For this review, take the finished solid that the model builds, in its own axes (mm). Coordinates: 2 decimals unless noted, no trailing zeros. Write each loop counter-clockwise with the first axis right and the second up, starting at its lowest first coordinate (ties: lowest second). Pieces come first, ordered by that corner, then holes. Notation, with made-up numbers: (23, -24) - (70, -24) arc R24 ccw to (70, 2) - close; hole circle Ø9 at (28, 35.5). An arc over 180 degrees is marked (long way). Write each question's results on one line, items separated by ' | '.
from build123d import *

# Parameters (mm, degrees)
SKIZZE1_R                       = 17.5
SKIZZE1_R_2                     = 2.2
SKIZZE1_R_3                     = 1.7
SKIZZE1_R_4                     = 2.05
AUFSATZ_LINEAR_AUSTRAGEN1_DEPTH = 2.5


with BuildPart() as part:
    # Skizze1 → Aufsatz-Linear austragen1 (new body)
    with BuildSketch(Plane.XY):
        with BuildLine():
            Line((9.914391914, -80), (9.914391914, 0))
            Line((9.914391914, 0), (9.914391914, 8))
            ThreePointArc((9.914391914, 8), (10.500178351, 9.414213562), (11.914391914, 10))
            Line((11.914391914, 10), (108.085608086, 10))
            ThreePointArc((108.085608086, 10), (109.499821649, 9.414213562), (110.085608086, 8))
            Line((110.085608086, 8), (110.085608086, 0))
            Line((110.085608086, 0), (110.085608086, -80))
            Line((110.085608086, -80), (110.085608086, -88))
            ThreePointArc((110.085608086, -88), (109.499821649, -89.414213562), (108.085608086, -90))
            Line((108.085608086, -90), (11.914391914, -90))
            ThreePointArc((11.914391914, -90), (10.500178351, -89.414213562), (9.914391914, -88))
            Line((9.914391914, -88), (9.914391914, -80))
        make_face()
        with Locations((60, -40)):
            Circle(SKIZZE1_R, mode=Mode.SUBTRACT)
        with Locations((35, -40)):
            Circle(SKIZZE1_R_2, mode=Mode.SUBTRACT)
        with Locations((50, -85)):
            Circle(SKIZZE1_R_3, mode=Mode.SUBTRACT)
        with Locations((24.914391914, -40)):
            Circle(SKIZZE1_R_4, mode=Mode.SUBTRACT)
        with Locations((40, -85)):
            Circle(SKIZZE1_R_3, mode=Mode.SUBTRACT)
        with Locations((95.085608086, -85)):
            Circle(SKIZZE1_R_3, mode=Mode.SUBTRACT)
        with Locations((24.914391914, -85)):
            Circle(SKIZZE1_R_3, mode=Mode.SUBTRACT)
        with Locations((14.914391914, -85)):
            Circle(SKIZZE1_R_3, mode=Mode.SUBTRACT)
        with Locations((105.085608086, -85)):
            Circle(SKIZZE1_R_3, mode=Mode.SUBTRACT)
        with Locations((40, 5)):
            Circle(SKIZZE1_R_3, mode=Mode.SUBTRACT)
        with Locations((50, 5)):
            Circle(SKIZZE1_R_3, mode=Mode.SUBTRACT)
        with Locations((70, 5)):
            Circle(SKIZZE1_R_3, mode=Mode.SUBTRACT)
        with Locations((80, 5)):
            Circle(SKIZZE1_R_3, mode=Mode.SUBTRACT)
        with Locations((95.085608086, 5)):
            Circle(SKIZZE1_R_3, mode=Mode.SUBTRACT)
        with Locations((105.085608086, 5)):
            Circle(SKIZZE1_R_3, mode=Mode.SUBTRACT)
        with Locations((80, -85)):
            Circle(SKIZZE1_R_3, mode=Mode.SUBTRACT)
        with Locations((95.085608086, -40)):
            Circle(SKIZZE1_R_4, mode=Mode.SUBTRACT)
        with Locations((70, -85)):
            Circle(SKIZZE1_R_3, mode=Mode.SUBTRACT)
        with Locations((85, -40)):
            Circle(SKIZZE1_R_2, mode=Mode.SUBTRACT)
        with Locations((24.914391914, 5)):
            Circle(SKIZZE1_R_3, mode=Mode.SUBTRACT)
        with Locations((14.914391914, 5)):
            Circle(SKIZZE1_R_3, mode=Mode.SUBTRACT)
        Polygon((101.462722804, -76.748846085), (103.274165445, -79.886356775), (106.897050727, -79.886356775), (108.708493369, -76.748846085), (106.897050727, -73.611335396), (103.274165445, -73.611335396), align=None, mode=Mode.SUBTRACT)
        Polygon((33.107285571, -56.381153914), (31.300179229, -53.251153914), (33.107285571, -50.121153914), (36.721498256, -50.121153914), (38.528604599, -53.251153914), (36.721498256, -56.381153914), align=None, mode=Mode.SUBTRACT)
        Polygon((18.537277196, -3.251153914), (16.725834555, -0.113643225), (13.102949273, -0.113643225), (11.291506631, -3.251153914), (13.102949273, -6.388664604), (16.725834555, -6.388664604), align=None, mode=Mode.SUBTRACT)
        Polygon((38.528604599, -3.251153914), (36.721498256, -0.121153914), (33.107285571, -0.121153914), (31.300179229, -3.251153914), (33.107285571, -6.381153914), (36.721498256, -6.381153914), align=None, mode=Mode.SUBTRACT)
        Polygon((18.528604599, -26.674423043), (16.721498256, -23.544423043), (13.107285571, -23.544423043), (11.300179229, -26.674423043), (13.107285571, -29.804423043), (16.721498256, -29.804423043), align=None, mode=Mode.SUBTRACT)
        Polygon((31.300179229, -26.748846085), (33.107285571, -29.878846085), (36.721498256, -29.878846085), (38.528604599, -26.748846085), (36.721498256, -23.618846085), (33.107285571, -23.618846085), align=None, mode=Mode.SUBTRACT)
        Polygon((16.721498256, -50.195576957), (18.528604599, -53.325576957), (16.721498256, -56.455576957), (13.107285571, -56.455576957), (11.300179229, -53.325576957), (13.107285571, -50.195576957), align=None, mode=Mode.SUBTRACT)
        Polygon((36.721498256, -73.618846085), (38.528604599, -76.748846085), (36.721498256, -79.878846085), (33.107285571, -79.878846085), (31.300179229, -76.748846085), (33.107285571, -73.618846085), align=None, mode=Mode.SUBTRACT)
        Polygon((16.725834555, -73.611335396), (18.537277196, -76.748846085), (16.725834555, -79.886356775), (13.102949273, -79.886356775), (11.291506631, -76.748846085), (13.102949273, -73.611335396), align=None, mode=Mode.SUBTRACT)
        Polygon((81.471395401, -76.748846085), (83.278501744, -79.878846085), (86.892714429, -79.878846085), (88.699820771, -76.748846085), (86.892714429, -73.618846085), (83.278501744, -73.618846085), align=None, mode=Mode.SUBTRACT)
        Polygon((101.471395401, -53.325576957), (103.278501744, -56.455576957), (106.892714429, -56.455576957), (108.699820771, -53.325576957), (106.892714429, -50.195576957), (103.278501744, -50.195576957), align=None, mode=Mode.SUBTRACT)
        Polygon((88.699820771, -53.251153914), (86.892714429, -50.121153914), (83.278501744, -50.121153914), (81.471395401, -53.251153914), (83.278501744, -56.381153914), (86.892714429, -56.381153914), align=None, mode=Mode.SUBTRACT)
        Polygon((86.892714429, -23.618846085), (88.699820771, -26.748846085), (86.892714429, -29.878846085), (83.278501744, -29.878846085), (81.471395401, -26.748846085), (83.278501744, -23.618846085), align=None, mode=Mode.SUBTRACT)
        Polygon((103.278501744, -29.804423043), (101.471395401, -26.674423043), (103.278501744, -23.544423043), (106.892714429, -23.544423043), (108.699820771, -26.674423043), (106.892714429, -29.804423043), align=None, mode=Mode.SUBTRACT)
        Polygon((83.278501744, -6.381153914), (81.471395401, -3.251153914), (83.278501744, -0.121153914), (86.892714429, -0.121153914), (88.699820771, -3.251153914), (86.892714429, -6.381153914), align=None, mode=Mode.SUBTRACT)
        Polygon((103.274165445, -6.388664604), (101.462722804, -3.251153914), (103.274165445, -0.113643225), (106.897050727, -0.113643225), (108.708493369, -3.251153914), (106.897050727, -6.388664604), align=None, mode=Mode.SUBTRACT)
    extrude(amount=AUFSATZ_LINEAR_AUSTRAGEN1_DEPTH)


solid = part.part
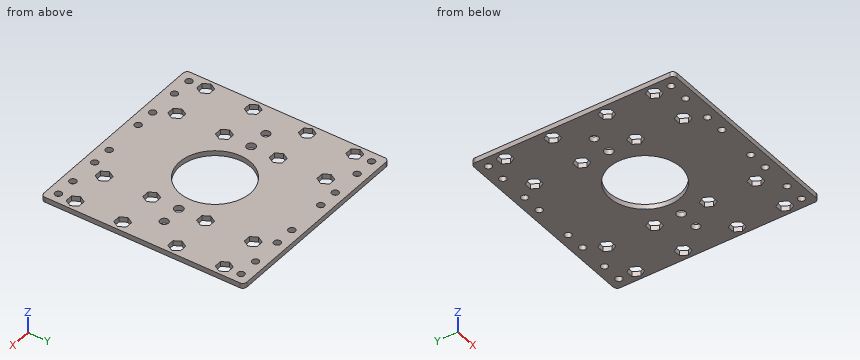
Q1. Take a section at D-D on x = 25. State the section outline as (y, z) points.
Results found:
outline: (-90, 0) - (-86.7, 0) - (-86.7, 2.5) - (-90, 2.5) - close; (-83.3, 0) - (-42.05, 0) - (-42.05, 2.5) - (-83.3, 2.5) - close; (-37.95, 0) - (3.3, 0) - (3.3, 2.5) - (-37.95, 2.5) - close; (6.7, 0) - (10, 0) - (10, 2.5) - (6.7, 2.5) - close
Q2. Take a section at B-B on x = 60. State the section outline as (y, z) points.
Results found:
outline: (-90, 0) - (-57.5, 0) - (-57.5, 2.5) - (-90, 2.5) - close; (-22.5, 0) - (10, 0) - (10, 2.5) - (-22.5, 2.5) - close
Q3. Take a section at A-A on y = -40. State the section outline as (x, z) points, plus the area to 3 significant figures.
Results found:
outline: (9.91, 0) - (22.86, 0) - (22.86, 2.5) - (9.91, 2.5) - close; (26.96, 0) - (32.8, 0) - (32.8, 2.5) - (26.96, 2.5) - close; (37.2, 0) - (42.5, 0) - (42.5, 2.5) - (37.2, 2.5) - close; (77.5, 0) - (82.8, 0) - (82.8, 2.5) - (77.5, 2.5) - close; (87.2, 0) - (93.04, 0) - (93.04, 2.5) - (87.2, 2.5) - close; (97.14, 0) - (110.09, 0) - (110.09, 2.5) - (97.14, 2.5) - close | area: 120 mm2
Q4. Take a section at C-C on x = 85. State the section outline as (y, z) points.
Results found:
outline: (-90, 0) - (-79.88, 0) - (-79.88, 2.5) - (-90, 2.5) - close; (-73.62, 0) - (-56.38, 0) - (-56.38, 2.5) - (-73.62, 2.5) - close; (-50.12, 0) - (-42.2, 0) - (-42.2, 2.5) - (-50.12, 2.5) - close; (-37.8, 0) - (-29.88, 0) - (-29.88, 2.5) - (-37.8, 2.5) - close; (-23.62, 0) - (-6.38, 0) - (-6.38, 2.5) - (-23.62, 2.5) - close; (-0.12, 0) - (10, 0) - (10, 2.5) - (-0.12, 2.5) - close
Q5. Wall thickness on line 1 along Y through (x, z) = (40, 1.85); line 2 along Y through (x, z) = (95, 1.1); line 3 along X through (y, z) = (-1.5, 0.25): over which ranges is each line inside the solid? List them lowest first. Write a range as from..to.
Results found:
line 1: -90..-86.7, -83.3..3.3, 6.7..10 | line 2: -90..-86.7, -83.3..-42.05, -37.95..3.3, 6.7..10 | line 3: 9.91..12.3, 17.53..32.31, 37.52..82.48, 87.69..102.47, 107.7..110.09
